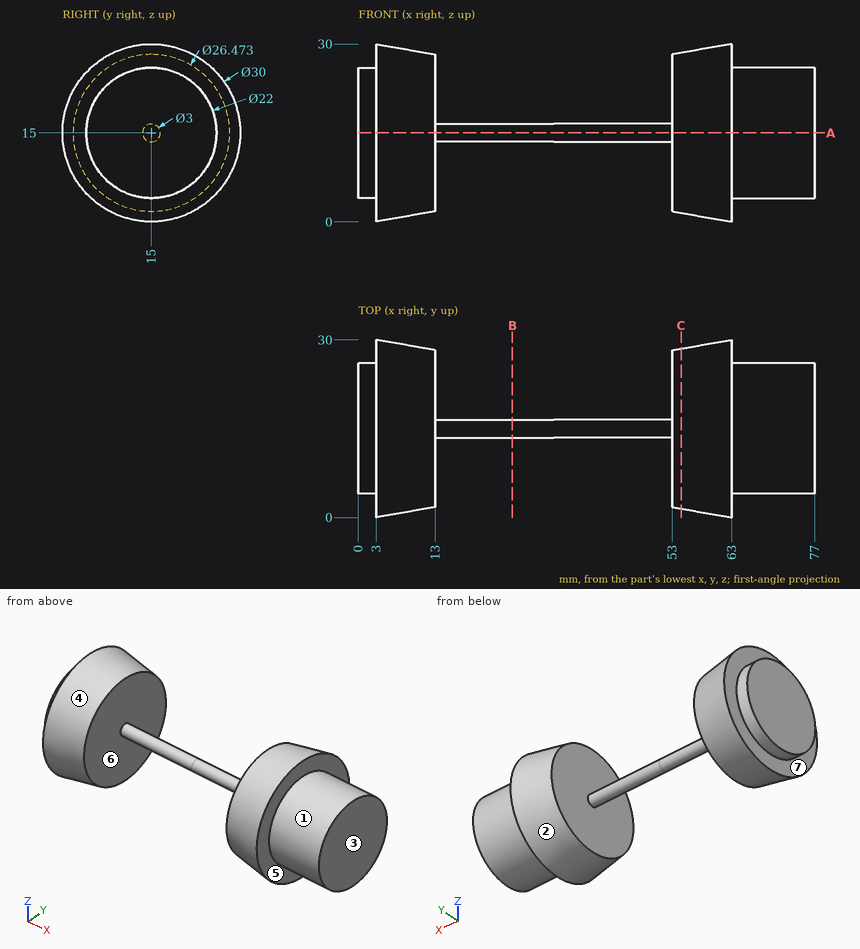
Can you work these out from the drawing? Everything is in mm from the part's minimum corner. A direction names the side the tool comes from. Round coordinates to 2 decimals unless told otherwise and drop trailing zeros. Loops run counter-clockwise (first coordinate to the right, second up) from the corner with the lowest first, then second, coordinate; pieces in that order, holes last. Notation, with made-up numbers: (88.25, -9) - (135.25, -9) arc R29 ccw to (135.25, 27) - close; hole circle Ø9 at (-13, 26.25). An arc over 180 degrees is marked (long way). Write item = value, one per line. Start each with the question number.
(1) If I drill on probe 1 along X at (y, z) = (3, 14); probe 2 along X at (y, z) = (23, 20); probe 3 along Y at (x, z) = (38.5, 15), over which ranges is the centre line in solid material (lowest first)? Write a range as [from, to].
(2) For the marked faces 1, 2 and 3, which set-ups out of +Z, -Z, +X, -X, +Y, -Y let a thin tool reach every point of the face, with its end or its side?
(3) If we section it at C-C (x = 54.5): Please give me the cut outline in (y, z).
(4) If we mould it in two halves opening along X, with no side actions, what happens to the marked faces 4, 5, 6 and 7? For each: released by +X, released by -X, zero draft, split by the parting line, or undercut.
(5) For P1, Ø8, axis at y = 10, z = 25, coming from the +X side; P2, Ø3, axis at x = 58, z = 17, coming from the +Y side; P3, Ø8, axis at x = 42, y = 22.5, coming from the +Z side; P4, Ø12, axis at x = 31.5, y = 16, coming from the -Z side, each with a flat end and sliding along its axis, tell me the tip position at first contact or that it passes through.
(6) If we section it at A-A (z = 15): Please give me the cut outline in (x, y), and give its area (3 significant figures).
(7) If we section it at B-B (x = 26): Please give me the cut outline in (y, z).
Ans:
q1.probe_1 = [3, 13], [53, 63]
q1.probe_2 = [0, 13], [53, 77]
q1.probe_3 = [13.5, 16.5]
q2.face_1 = +X
q2.face_2 = none
q2.face_3 = +Z, -Z, +X, +Y, -Y
q3.outline = circle Ø27 at (15, 15)
q4.face_4 = undercut
q4.face_5 = released by +X
q4.face_6 = undercut
q4.face_7 = released by -X
q5.P1 = 77
q5.P2 = 29.29
q5.P3 = through
q5.P4 = 13.5
q6.outline = (0, 4) - (3, 4) - (3, 0) - (13, 1.76) - (13, 13.5) - (53, 13.5) - (53, 1.76) - (63, 0) - (63, 4) - (77, 4) - (77, 26) - (63, 26) - (63, 30) - (53, 28.24) - (53, 16.5) - (13, 16.5) - (13, 28.24) - (3, 30) - (3, 26) - (0, 26) - close
q6.area = 1,060 mm²
q7.outline = circle Ø3 at (15, 15)
